Read the model definition and answer for the solid it produces. Units are mm, in the model's axes. A direction names the side the tool comes from. Give positions to 0.01 mm unless a question says otherwise; leave off trailing zeros. Order: outer loops, then holes, each group sorted by start corner. A loop starts at its lowest first (then second) coordinate and runs counter-clockwise, first axis right, second up. Notation, with made-up numbers: M 58.5,87 L 101.5,87 A16 ccw 101.5,97 Z; hole C 73.5,-11 d2. An arc over 180 degrees is marked long. One line per item, written item: value.
from build123d import *

# Parameters (mm, degrees)
F0_W     = 88.9
F0_H     = 127
F1_DEPTH = 76.2
F0_W_2   = 76.2
F0_H_2   = 4.0558092296
F0_H_3   = 3.3183873165
F0_H_4   = 2.9496774077
F2_DEPTH = 71.12
F0_H_5   = 27.6327425224
F0_H_6   = 26.1783864116
F0_H_7   = 23.7817749148
F0_H_8   = 28.9232221973
F3_DEPTH = 6.35


with BuildPart() as f1:
    # F0 (on Front) → F1 (new body)
    with BuildSketch(Plane.XZ):
        with Locations((1.440508941, 0)):
            Rectangle(F0_W, F0_H)
        Polygon((-36.659491059, 58.42), (39.540508941, 58.42), (39.540508941, 30.7872574776), (39.540508941, 27.8375800699), (39.540508941, 1.6591936583), (39.540508941, -1.6591936583), (39.540508941, -25.4409685731), (39.540508941, -29.4967778027), (39.540508941, -58.42), (-36.659491059, -58.42), (-36.659491059, -29.4967778027), (-36.659491059, -25.4409685731), (-36.659491059, -1.6591936583), (-36.659491059, 1.6591936583), (-36.659491059, 27.8375800699), (-36.659491059, 30.7872574776), align=None, mode=Mode.SUBTRACT)
    extrude(amount=F1_DEPTH)

    # F0 (on Front) → F2 (join)
    with BuildSketch(Plane.XZ):
        with Locations((1.440508941, -27.4688731879)):
            Rectangle(F0_W_2, F0_H_2)
        with Locations((1.440508941, 0)):
            Rectangle(F0_W_2, F0_H_3)
        with Locations((1.440508941, 29.3124187738)):
            Rectangle(F0_W_2, F0_H_4)
    extrude(amount=F2_DEPTH)

    # F0 (on Front) → F3 (join)
    with BuildSketch(Plane.XZ):
        with Locations((1.440508941, 44.6036287388)):
            Rectangle(F0_W_2, F0_H_5)
        with Locations((1.440508941, 14.7483868641)):
            Rectangle(F0_W_2, F0_H_6)
        with Locations((1.440508941, -13.5500811157)):
            Rectangle(F0_W_2, F0_H_7)
        with Locations((1.440508941, -43.9583889014)):
            Rectangle(F0_W_2, F0_H_8)
    extrude(amount=F3_DEPTH)


solid = f1.part
1) Find section C-C, the plane x = 11. Write down the section's boundary in (y, z), plus the area to 3 significant figures.
Reported:
outline: M -76.2,-63.5 L 0,-63.5 L 0,63.5 L -76.2,63.5 L -76.2,58.42 L -6.35,58.42 L -6.35,30.79 L -71.12,30.79 L -71.12,27.84 L -6.35,27.84 L -6.35,1.66 L -71.12,1.66 L -71.12,-1.66 L -6.35,-1.66 L -6.35,-25.44 L -71.12,-25.44 L -71.12,-29.5 L -6.35,-29.5 L -6.35,-58.42 L -76.2,-58.42 Z
area: 2,180 mm^2
2) Which of the six approach directions +Z, -Z, +X, -X, +Y, -Y give full straight-line access (tool end or side, diameter ignored) to faces 1 (the face through (1, -6.35, 15)), 2 (the face through (-43.009, -38, -1))?
Reported:
face 1: -Y
face 2: +Z, -Z, -X, +Y, -Y
3) Find section A-A, the plane y = -61.5. Write down the section's boundary in (x, z).
Reported:
outline: M -43.01,-63.5 L 45.89,-63.5 L 45.89,63.5 L -43.01,63.5 Z; hole M -36.66,-58.42 L 39.54,-58.42 L 39.54,-29.5 L -36.66,-29.5 Z; hole M -36.66,-25.44 L 39.54,-25.44 L 39.54,-1.66 L -36.66,-1.66 Z; hole M -36.66,1.66 L 39.54,1.66 L 39.54,27.84 L -36.66,27.84 Z; hole M -36.66,30.79 L 39.54,30.79 L 39.54,58.42 L -36.66,58.42 Z
4) Find section B-B, the plane z = -14. Write down the section's boundary in (x, y).
Reported:
outline: M -43.01,-76.2 L -36.66,-76.2 L -36.66,-6.35 L 39.54,-6.35 L 39.54,-76.2 L 45.89,-76.2 L 45.89,0 L -43.01,0 Z
5) Each of these flat-tipped pins is pushed along its axis until it touches: pin 1 Ø2.5 at (x, z) = (-15, -0.5) entering from -Y; pin 2 Ø1 at (x, z) = (-1, -39.5) entering from -Y. Where does it stop, or does it pass through?
Reported:
pin 1: stops at y = -71.12
pin 2: stops at y = -6.35
6) Determine the mould class of faces 3 (the face through (-38, -76.2, 5)), 4 (the face through (1, -38, -1.659)), 5 (the face through (45.891, -38, -1)) for opening direction X: +X half, -X half, draft (parallel to the pull), parting line (faces both ways), or undercut.
Reported:
face 3: draft
face 4: undercut
face 5: +X half
7) Consider probe 1 along Z at (x, y) = (3, -61.5); probe 2 along X at (y, z) = (-33.5, 36.5); probe 3 along Y at (x, z) = (-24, 21). Determine where each line is inside the solid, lowest interval first.
Reported:
probe 1: z = -63.5 to -58.42, -29.5 to -25.44, -1.66 to 1.66, 27.84 to 30.79, 58.42 to 63.5
probe 2: x = -43.01 to -36.66, 39.54 to 45.89
probe 3: y = -6.35 to 0
